```python
from build123d import *

# Parameters (mm, degrees)
CROQUIS1_W              = 35
CROQUIS1_H              = 29.5
SALIENTE_EXTRUIR1_DEPTH = 2
SALIENTE_EXTRUIR2_DEPTH = 1.6
CROQUIS3_R              = 4
SALIENTE_EXTRUIR3_DEPTH = 3.7
CROQUIS4_W              = 5.5
CROQUIS4_H              = 1.8
CROQUIS4_W_2            = 5
SALIENTE_EXTRUIR4_DEPTH = 12
CROQUIS5_W              = 1
CROQUIS5_H              = 20
CORTAR_EXTRUIR1_DEPTH   = 29.118543703
CROQUIS6_R              = 0.500490027
CORTAR_EXTRUIR2_DEPTH   = 12
REDONDEO1_R             = 1
SALIENTE_EXTRUIR5_START = 1.6
SALIENTE_EXTRUIR5_DEPTH = 1.6


with BuildPart() as part:
    # Croquis1 → Saliente-Extruir1 (new body)
    with BuildSketch(Plane(origin=(0, 0, 0), x_dir=(1, 0, 0), z_dir=(0, 1, 0))):
        Rectangle(CROQUIS1_W, CROQUIS1_H)
    extrude(amount=SALIENTE_EXTRUIR1_DEPTH)

    # Croquis2 → Saliente-Extruir2 (add)
    with BuildSketch(Plane.XY.offset(14.75)):
        with BuildLine():
            Line((14.1, 2), (-3.9, 2))
            Line((-3.9, 2), (2.207935866, 10.043820198))
            ThreePointArc((2.207935866, 10.043820198), (5.1, 11.5), (7.992064134, 10.043820198))
            Line((7.992064134, 10.043820198), (14.1, 2))
        make_face()
    extrude(amount=-SALIENTE_EXTRUIR2_DEPTH)

    # Croquis3 → Saliente-Extruir3 (add)
    with BuildSketch(Plane.XY.offset(14.75)):
        with Locations(Location((3.7, 8.1, 0), (0, 0, 196.564510331))):
            Circle(CROQUIS3_R)
    extrude(amount=SALIENTE_EXTRUIR3_DEPTH)

    # Croquis4 → Saliente-Extruir4 (add)
    with BuildSketch(Plane(origin=(0, 2, 0), x_dir=(1, 0, 0), z_dir=(0, 1, 0))):
        with Locations((-14.75, 3.15)):
            Rectangle(CROQUIS4_W, CROQUIS4_H)
        with Locations((12.5, 3.15)):
            Rectangle(CROQUIS4_W_2, CROQUIS4_H)
    extrude(amount=SALIENTE_EXTRUIR4_DEPTH)

    # Croquis5 → Cortar-Extruir1 (cut, through all)
    with BuildSketch(Plane(origin=(0, 2, 0), x_dir=(1, 0, 0), z_dir=(0, 1, 0))):
        with Locations((15.5, 0)):
            Rectangle(CROQUIS5_W, CROQUIS5_H)
    extrude(amount=-CORTAR_EXTRUIR1_DEPTH, mode=Mode.SUBTRACT)

    # Croquis6 → Cortar-Extruir2 (cut)
    with BuildSketch(Plane.XZ):
        with Locations(Location((-8.5, -10, 0), (0, 0, 270))):
            Circle(CROQUIS6_R)
        with Locations(Location((-2.5, -10, 0), (0, 0, 270))):
            Circle(CROQUIS6_R)
        with Locations(Location((3.5, -10, 0), (0, 0, 270))):
            Circle(CROQUIS6_R)
        with Locations(Location((9.5, -10, 0), (0, 0, 270))):
            Circle(CROQUIS6_R)
        with Locations(Location((-2.5, 10, 0), (0, 0, 270))):
            Circle(CROQUIS6_R)
        with Locations(Location((3.5, 10, 0), (0, 0, 270))):
            Circle(CROQUIS6_R)
        with Locations(Location((9.5, 10, 0), (0, 0, 270))):
            Circle(CROQUIS6_R)
        with Locations(Location((-8.5, 10, 0), (0, 0, 270))):
            Circle(CROQUIS6_R)
    extrude(amount=-CORTAR_EXTRUIR2_DEPTH, mode=Mode.SUBTRACT)

    # Redondeo1
    redondeo1_edges = [part.edges().sort_by_distance(p)[0] for p in [
        (17.5, 1, 14.75),
        (-17.5, 1, 14.75),
        (-17.5, 1, -14.75),
        (17.5, 1, -14.75),
    ]]
    fillet(redondeo1_edges, radius=REDONDEO1_R)

    # Croquis7 → Saliente-Extruir5 (add)
    with BuildSketch(Plane(origin=(0, 0, 14.75), x_dir=(-1, 0, 0), z_dir=(0, 0, -1)).offset(SALIENTE_EXTRUIR5_START)):
        with BuildLine():
            Line((3.9, 2), (-0.052229294, 9.741270508))
            ThreePointArc((-0.052229294, 9.741270508), (-2.499470939, 11.915590383), (-5.750816337, 11.534261544))
            Line((-5.750816337, 11.534261544), (-5.750816337, 2))
            Line((-5.750816337, 2), (3.9, 2))
        make_face()
    extrude(amount=-SALIENTE_EXTRUIR5_DEPTH)


solid = part.part
```
Geometry check sheet. Reference: the model listing, model coordinates, mm. A direction names the side the tool comes from. Give positions to 0.01 mm unless a question says otherwise; leave off trailing zeros. Loops run counter-clockwise (first coordinate to the right, second up) from the corner with the lowest first, then second, coordinate; pieces in that order, holes last. Notation, with made-up numbers: M -25.75,66 L -12.75,66 A13 ccw -12.75,78 Z; hole C 13,37.5 d7. An arc over 180 degrees is marked long. Write item = value, one per line.
(1) Tool access check on faces 1 (the face through (12, 14, -3)), 2 (the face through (12, 8, -2.25)), 3 (the face through (15, 1.8, -1.4)), 4 (the face through (-15, 8, -4.05)), 5 (the face through (10, 8, -3)). Record the directions out of +Z, -Z, +X, -X, +Y, -Y that give a thin tool (end or side, any length) a straight path to the whole face; none if there is none.
Answer below:
face_1 = +Z, -Z, +X, -X, +Y
face_2 = +X, -X, +Y
face_3 = +Y, -Y
face_4 = -Z, +X, -X, +Y
face_5 = -Z, +Y
(2) Sectioned sample at A-A, the plane x = -8.5. Record the cut outline in (y, z), plus the area to 3 significant figures.
Answer below:
outline = M 0,-14.75 L 2,-14.75 L 2,-10.5 L 0,-10.5 Z; M 0,-9.5 L 2,-9.5 L 2,9.5 L 0,9.5 Z; M 0,10.5 L 2,10.5 L 2,14.75 L 0,14.75 Z
area = 55.0 mm2
(3) Sectioned sample at D-D, the plane x = 15.5. Record the cut outline in (y, z).
Answer below:
outline = M 0,-14.75 L 2,-14.75 L 2,-10 L 0,-10 Z; M 0,10 L 2,10 L 2,14.75 L 0,14.75 Z
(4) Gauge pin test, flat ends, axial feed: pin 1 Ø4 at (x, y) = (12.5, 9) entering from -Z; pin 2 Ø3 at (x, y) = (11.5, 3) entering from +Z; pin 3 Ø0.9 at (x, z) = (3.5, 10) entering from -Y; pin 4 Ø2 at (y, z) = (9.5, 13.5) entering from -X. Record the tip position at first contact, or that the pin passes through.
Answer below:
pin_1 = -4.05
pin_2 = 14.75
pin_3 = through
pin_4 = -0.58
(5) Release check for a two-part mould opening along X. For faces 6 (the face through (17.5, 1, 0)), 7 (the face through (-17.5, 1.8, -1)), 8 (the face through (-3, 1, -10)), 9 (the face through (0, 0, 0)) record: released by +X, released by -X, zero draft, split by the parting line, or undercut.
Answer below:
face_6 = released by +X
face_7 = released by -X
face_8 = undercut
face_9 = zero draft
(6) Material ranges on line 1 (X direction, y = 1.5, z = -6.5); line 2 (X direction, y = 6.75, z = -3.5); line 3 (Z direction, x = -15, y = 9.25), recorded low to high. Write a range as [from, to].
Answer below:
line_1 = [-17.5, 15], [16, 17.5]
line_2 = [-17.5, -12], [10, 15]
line_3 = [-4.05, -2.25]
(7) Sectioned sample at B-B, the plane z = -3. Record the cut outline in (x, y), plus the area to 3 significant figures.
Answer below:
outline = M -17.5,0 L 15,0 L 15,14 L 10,14 L 10,2 L -12,2 L -12,14 L -17.5,14 Z; M 16,0 L 17.5,0 L 17.5,2 L 16,2 Z
area = 194 mm2
(8) Sectioned sample at C-C, the plane y = 12.75. Record the cut outline in (x, z).
Answer below:
outline = M -17.5,-4.05 L -12,-4.05 L -12,-2.25 L -17.5,-2.25 Z; M 10,-4.05 L 15,-4.05 L 15,-2.25 L 10,-2.25 Z
